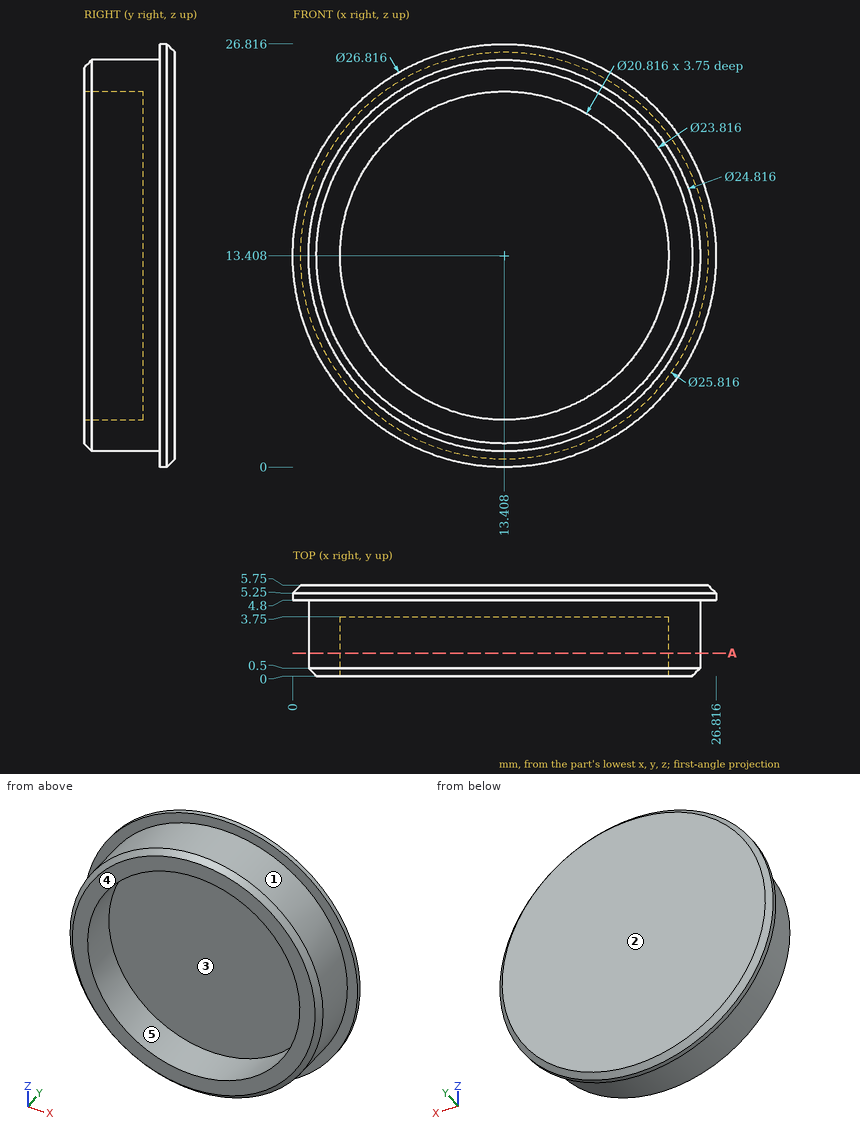
Study the drawing (mm; zero at the part's minimum x, y, z) and answer. A direction names the side the tool comes from. Coordinates: 2 decimals unless noted, no trailing zeros. Write each loop counter-clockwise with the first axis right and the second up, starting at its lowest first coordinate (ties: lowest second). Pieces come first, ordered by that corner, then holes. Notation, with made-up numbers: M 37.5,82.25 L 59.5,82.25 A13 ccw 59.5,87.25 Z; hole C 80.25,43 d4. An arc over 180 degrees is marked long. Use a Markdown table: item, result. Add a question column.
1. Which of the six approach directions +Z, -Z, +X, -X, +Y, -Y give full straight-line access (tool end or side, diameter ignored) to the marked faces 4 and 5?
2. Section A-A (y = 1.45) is taken. Give the vertices of the cut face in (x, z), plus the area to 3 significant figures.
3. Given P1, Ø1.5, axis at y = 4, z = 21, coming from the -X side; P2, Ø3, axis at x = 20.5, y = 4.5, coming from the +Z side; P3, Ø3, axis at y = 4, z = 19, coming from the -X side, each flat-ended and moving along its own axis, determine where each tip first touches the part or whether it passes through.
4. For a pull along X with two mould halves and no side action, classify the marked faces 1, 2 and 3 as +X half, -X half, draft (parallel to the pull), parting line (faces both ways), or undercut.
5. Straight lines are drawn through the part: line 1 along Y through (x, z) = (23.25, 16); line 2 along Z through (x, y) = (6.75, 2.85); line 3 along Z through (x, y) = (22.25, 3.7). For each, find the intervals that lie inside material, in ascending order. Write a range as [from, to].
Data:
| question | item | result |
|---|---|---|
| 1 | face 4 | +Z, -Z, +X, -X, -Y |
| 1 | face 5 | -Y |
| 2 | outline | C 13.41,13.41 d24.82; hole C 13.41,13.41 d20.82 |
| 2 | area | 143 mm2 |
| 3 | P1 | stops at x = 3.06 |
| 3 | P2 | stops at z = 25.58 |
| 3 | P3 | stops at x = 0.72 |
| 4 | face 1 | parting line |
| 4 | face 2 | draft |
| 4 | face 3 | undercut |
| 5 | line 1 | y = [3.75, 5.75] |
| 5 | line 2 | z = [2.94, 5.41], [21.41, 23.88] |
| 5 | line 3 | z = [4.7, 7.92], [18.9, 22.11] |
